Geometry: final body of the model. Coordinates: model frame, mm. Round coordinates to 2 decimals unless told otherwise and drop trailing zeros. Order: outer loops, then holes, each group sorted by start corner. A loop starts at its lowest first (then second) coordinate and runs counter-clockwise, first axis right, second up. Notation, with made-up numbers: M 9.25,-4 L 32.25,-4 A20 cw 32.25,22 Z; hole C 40.25,12 d1. An arc over 180 degrees is marked long. Return JSON: item names as keys, results as strings. Group by question number.
Q1. Cut plane A-A on y = 12.7. Output: boundary loops of the cut face in (x, z).
Q2. Cut plane D-D on y = 2.75. Output: boundary loops of the cut face in (x, z).
Q3. Contact query for a flat-ended pin moving along its axis: pin 1 (6 mm diameter, centred on y = 12.5, z = -5.5, fed in from +X). Output: stop coordinate, or through.
Q4. Cut plane B-B on x = -0.6. Output: boundary loops of the cut face in (y, z), and give its area (3 significant figures).
Q5. Ray query, probe 1 along Z at (x, y) = (-0.05, 10.25); probe 2 along Y at (x, z) = (-0.2, -24.5); probe 3 along Z at (x, y) = (-0.9, 19). Return the intervals inside material, ascending.
Q6. Cut plane C-C on z = -14. Output: boundary loops of the cut face in (x, y), and give its area (3 significant figures).
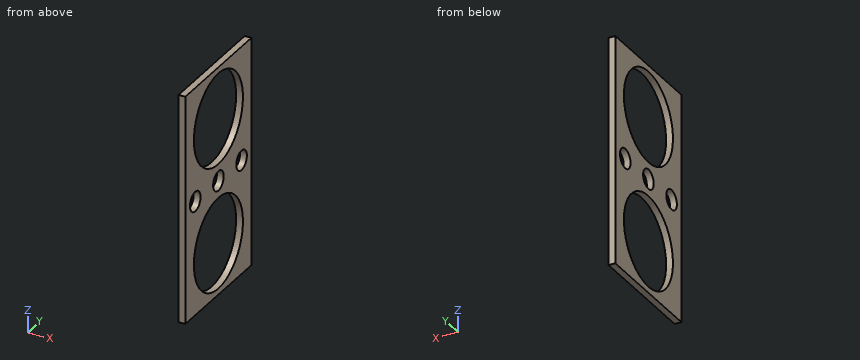
```python
from build123d import *

# Parameters (mm, degrees)
SKETCH2_W           = 47.13986
SKETCH2_H           = 25.4
SKETCH2_R           = 2.032
SKETCH2_R_2         = 9.411008891
BOSS_EXTRUDE1_DEPTH = 1.41224


with BuildPart() as part:
    # Sketch2 → Boss-Extrude1 (new body)
    with BuildSketch(Plane(origin=(0, 0, 0), x_dir=(0, 0, -1), z_dir=(1, 0, 0))):
        with Locations((23.56993, 12.7)):
            Rectangle(SKETCH2_W, SKETCH2_H)
        with Locations((23.56993, 21.59)):
            Circle(SKETCH2_R, mode=Mode.SUBTRACT)
        with Locations((23.56993, 12.7)):
            Circle(SKETCH2_R, mode=Mode.SUBTRACT)
        with Locations((23.56993, 3.81)):
            Circle(SKETCH2_R, mode=Mode.SUBTRACT)
        with Locations((10.668, 12.7)):
            Circle(SKETCH2_R_2, mode=Mode.SUBTRACT)
        with Locations(Location((36.47186, 12.7, 0), (0, 0, 180))):
            Circle(SKETCH2_R_2, mode=Mode.SUBTRACT)
    extrude(amount=-BOSS_EXTRUDE1_DEPTH)


solid = part.part
```
Result sheet:
{
 "1": {"outline": "M -1.41,-47.14 L 0,-47.14 L 0,-45.88 L -1.41,-45.88 Z; M -1.41,-27.06 L 0,-27.06 L 0,-25.6 L -1.41,-25.6 Z; M -1.41,-21.54 L 0,-21.54 L 0,-20.08 L -1.41,-20.08 Z; M -1.41,-1.26 L 0,-1.26 L 0,0 L -1.41,0 Z"},
 "2": {"outline": "M -1.41,-47.14 L 0,-47.14 L 0,-25.3 L -1.41,-25.3 Z; M -1.41,-21.84 L 0,-21.84 L 0,0 L -1.41,0 Z"},
 "3": {"pin 1": "passes through"},
 "4": {"outline": "M 0,-47.14 L 25.4,-47.14 L 25.4,0 L 0,0 Z; hole C 3.81,-23.57 d4.06; hole C 12.7,-36.47 d18.82; hole C 12.7,-10.67 d18.82; hole C 12.7,-23.57 d4.06; hole C 21.59,-23.57 d4.06", "area": "602 mm²"},
 "5": {"probe 1": "z = -47.14 to -45.56, -27.39 to -19.75, -1.58 to 0", "probe 2": "y = 0 to 2, 5.62 to 10.89, 14.51 to 19.78, 23.4 to 25.4", "probe 3": "z = -47.14 to -43.46, -29.48 to -17.66, -3.68 to 0"},
 "6": {"outline": "M -1.41,0 L 0,0 L 0,3.9 L -1.41,3.9 Z; M -1.41,21.5 L 0,21.5 L 0,25.4 L -1.41,25.4 Z", "area": "11.0 mm²"}
}
